Build history of the part. All positions in model axes, mm. A direction names the side the tool comes from. Round coordinates to 2 decimals unless told otherwise and drop trailing zeros. Write each loop counter-clockwise with the first axis right and the second up, starting at its lowest first coordinate (ties: lowest second). Pieces come first, ordered by that corner, then holes. Notation, with made-up numbers: (26.25, 88) -> (36.25, 88) arc R24 cw to (36.25, 105) -> close; hole circle Ø6 at (58.25, 72). An arc over 180 degrees is marked (long way). Return JSON: item names as keys, results as strings.
from build123d import *

# Parameters (mm, degrees)
SKETCH1_R           = 17
BOSS_EXTRUDE1_DEPTH = 10
SKETCH2_R           = 10.475
BOSS_EXTRUDE2_DEPTH = 12
FILLET1_R           = 2
SKETCH3_R           = 32.5
BOSS_EXTRUDE3_DEPTH = 10
SKETCH4_R           = 3
CUT_EXTRUDE1_DEPTH  = 57.004464108


with BuildPart() as part:
    # Sketch1 → Boss-Extrude1 (new body)
    with BuildSketch(Plane.XY):
        Circle(SKETCH1_R)
    extrude(amount=BOSS_EXTRUDE1_DEPTH)

    # Sketch2 → Boss-Extrude2 (add)
    with BuildSketch(Plane.XY.offset(10)):
        Circle(SKETCH2_R)
    extrude(amount=BOSS_EXTRUDE2_DEPTH)

    # Fillet1
    fillet1_edges = [part.edges().sort_by_distance(p)[0] for p in [
        (-17, 0, 10),
        (-10.475, 0, 22),
    ]]
    fillet(fillet1_edges, radius=FILLET1_R)

    # Sketch3 → Boss-Extrude3 (add)
    with BuildSketch(Plane(origin=(0, 0, 0), x_dir=(-1, 0, 0), z_dir=(0, 0, -1))):
        Circle(SKETCH3_R)
    extrude(amount=BOSS_EXTRUDE3_DEPTH)

    # Sketch4 → Cut-Extrude1 (cut, through all)
    with BuildSketch(Plane(origin=(0, 0, -10), x_dir=(-1, 0, 0), z_dir=(0, 0, -1))):
        with Locations((26, 0)):
            Circle(SKETCH4_R)
        with Locations((13, -22.516660498)):
            Circle(SKETCH4_R)
        with Locations((-13, -22.516660498)):
            Circle(SKETCH4_R)
        with Locations((-26, 0)):
            Circle(SKETCH4_R)
        with Locations((-13, 22.516660498)):
            Circle(SKETCH4_R)
        with Locations((13, 22.516660498)):
            Circle(SKETCH4_R)
    extrude(amount=-CUT_EXTRUDE1_DEPTH, mode=Mode.SUBTRACT)


solid = part.part
Q1. 3-axis set-ups, long thin cutter, end or side, ignore diameter. For faces 4 (the cylindrical face through (15.21, -20.49, -5.07)), 5 (the cylindrical face through (9.139, 14.334, 3.944)): which of +Z, -Z, +X, -X, +Y, -Y reach the whole face in a straight line?
Verdict:
{"face 4": "+Z, -Z", "face 5": "+Z"}
Q2. Saw through at A-A on y = 0. List the corners of the cut face in (x, z) (3 decimals), then the cut area to 3 significant figures.
Verdict:
{"outline": "(-32.5, -10) -> (-29, -10) -> (-29, 0) -> (-32.5, 0) -> close; (-23, -10) -> (23, -10) -> (23, 0) -> (17, 0) -> (17, 8) arc R2 ccw to (15, 10) -> (10.475, 10) -> (10.475, 20) arc R2 ccw to (8.475, 22) -> (-8.475, 22) arc R2 ccw to (-10.475, 20) -> (-10.475, 10) -> (-15, 10) arc R2 ccw to (-17, 8) -> (-17, 0) -> (-23, 0) -> close; (29, -10) -> (32.5, -10) -> (32.5, 0) -> (29, 0) -> close", "area": "1,120 mm²"}
Q3. Saw through at D-D on z = 6. List the corners of the cut face in (x, y), then the cut area to 3 significant figures.
Verdict:
{"outline": "circle Ø34 at (0, 0)", "area": "908 mm²"}
Q4. Saw through at C-C on x = 0. List the corners of the cut face in (y, z) (3 decimals), then the cut area to 3 significant figures.
Verdict:
{"outline": "(-32.5, -10) -> (32.5, -10) -> (32.5, 0) -> (17, 0) -> (17, 8) arc R2 ccw to (15, 10) -> (10.475, 10) -> (10.475, 20) arc R2 ccw to (8.475, 22) -> (-8.475, 22) arc R2 ccw to (-10.475, 20) -> (-10.475, 10) -> (-15, 10) arc R2 ccw to (-17, 8) -> (-17, 0) -> (-32.5, 0) -> close", "area": "1,240 mm²"}
Q5. Two-plate mould, pull along X, no slides. Class faces 1 (the cylindrical face through (15.38, 20.69, -5.07)), 2 (the cylindrical face through (4.834, -9.293, 14.93)), 3 (the flat face through (-14, -14, 0)): +X half, -X half, draft (parallel to the pull), parting line (faces both ways), or undercut.
Verdict:
{"face 1": "undercut", "face 2": "parting line", "face 3": "draft"}
Q6. Pin check, flat tips, straight feed: pin 1 Ø1 at (x, y) = (-19.5, -10) entering from +Z; pin 2 Ø12 at (x, y) = (-17.5, -5) entering from +Z; pin 3 Ø5 at (y, z) = (10.5, 1.5) entering from -X; pin 4 Ø3.5 at (x, y) = (-13, 22.52) entering from +Z. Stop position of each tip, or through.
Verdict:
{"pin 1": "stops at z = 0", "pin 2": "stops at z = 10", "pin 3": "stops at x = -31.37", "pin 4": "passes through"}
Q7. Wall check: L1, parallel to Y at x = -13, z = -4.25; L2, parallel to X at y = 22, z = -7; L3, parallel to X at y = -0.5, z = 11.5. Give the ranges that are in metal, low to high.
Verdict:
{"L1": "y = -29.79 to -25.52, -19.52 to 19.52, 25.52 to 29.79", "L2": "x = -23.92 to -15.96, -10.04 to 10.04, 15.96 to 23.92", "L3": "x = -10.46 to 10.46"}
Q8. Saw through at B-B on x = 26. List the corners of the cut face in (y, z), then the cut area to 3 significant figures.
Verdict:
{"outline": "(-19.5, -10) -> (-3, -10) -> (-3, 0) -> (-19.5, 0) -> close; (3, -10) -> (19.5, -10) -> (19.5, 0) -> (3, 0) -> close", "area": "330 mm²"}
